Answer from the drawing. Dimensions are ordinates in mm from the lowest x, y and z of the part. A direction names the side the tool comes from. Round coordinates to 2 decimals unless told otherwise and drop trailing zeros. Order: outer loops, then holes, each group sorted by start corner. A loop starts at its lowest first (then second) coordinate and runs counter-clockwise, first axis right, second up. Notation, with made-up numbers: (26.25, 36) -> (85.25, 36) arc R17 ccw to (85.25, 63) -> close; hole circle Ø11 at (4.25, 57.25). An arc over 180 degrees is marked (long way). Use a Markdown table: item, result. Add a question column.
1. For the marked faces 1 and 2, determine the directions among +Z, -Z, +X, -X, +Y, -Y from which every point of the face is accessible in a straight line to the end or side of a thin tool.
2. Section B-B, the plane z = 25.5 is taken. Give the vertices of the cut face in (x, y), then the cut area to 3 significant figures.
3. Section C-C, the plane x = 11 is taken. Give the vertices of the cut face in (y, z).
4. Section A-A, the plane y = 1.25 is taken. Give the vertices of the cut face in (x, z).
5. Consider L1, parallel to X at y = 0.5, z = 14; L2, parallel to Y at x = 8.75, z = 23. Determine where each line is inside the solid, lowest interval first. Write a range as [from, to].
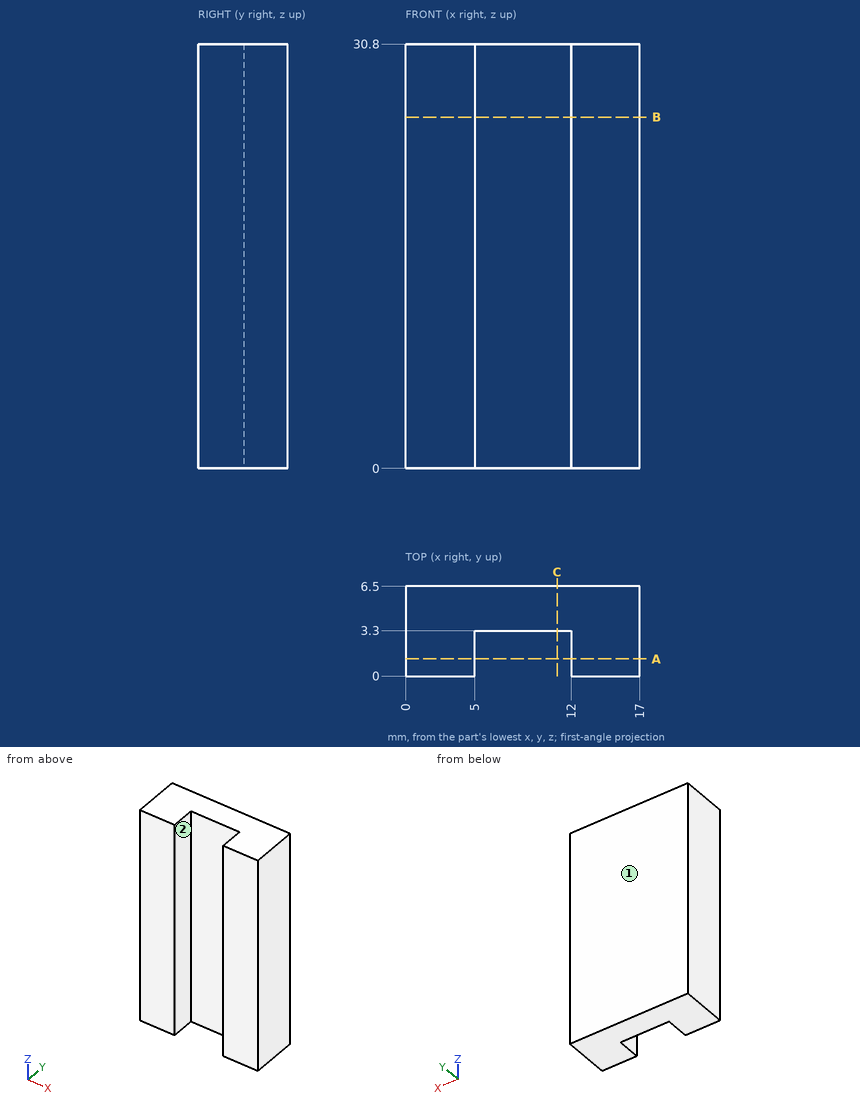
Verdict:
| question | item | result |
|---|---|---|
| 1 | face 1 | +Z, -Z, +X, -X, +Y |
| 1 | face 2 | +Z, -Z, -Y |
| 2 | outline | (0, 0) -> (5, 0) -> (5, 3.3) -> (12, 3.3) -> (12, 0) -> (17, 0) -> (17, 6.5) -> (0, 6.5) -> close |
| 2 | area | 87.4 mm2 |
| 3 | outline | (3.3, 0) -> (6.5, 0) -> (6.5, 30.8) -> (3.3, 30.8) -> close |
| 4 | outline | (0, 0) -> (5, 0) -> (5, 30.8) -> (0, 30.8) -> close; (12, 0) -> (17, 0) -> (17, 30.8) -> (12, 30.8) -> close |
| 5 | L1 | x = [0, 5], [12, 17] |
| 5 | L2 | y = [3.3, 6.5] |
